For this review, take the finished solid that the model builds, in its own axes (mm). Round coordinates to 2 decimals unless told otherwise and drop trailing zeros. Loops run counter-clockwise (first coordinate to the right, second up) from the corner with the lowest first, then second, coordinate; pieces in that order, holes last. Notation, with made-up numbers: (80.25, 6.5) -> (118.25, 6.5) arc R20 ccw to (118.25, 39.5) -> close; hole circle Ø5 at (72, 47.25). An arc over 180 degrees is marked (long way). Write each question's results on one line, items separated by ' | '.
Autodesk Inventor part; units mm, degrees
ref_plane "YZ Plane" through (0, 0, 0) normal (1, 0, 0) x (0, 1, 0)
ref_plane "XZ Plane" through (0, 0, 0) normal (0, 1, 0) x (-1, 0, 0)
ref_plane "XY Plane" through (0, 0, 0) normal (0, 0, 1) x (1, 0, 0)
sketch "Sketch1" plane through (0, 0, 0) normal (0, 1, 0) x (-1, 0, 0)
  line L0 (0, 0) -> (31, 0)
  line L1 (31, 0) -> (31, -84)
  line L2 (31, -84) -> (0, -84)
  line L3 (0, -84) -> (0, 0)
  line L4 (31, -42) -> (0, -42)
  circle A0 centre (20.5, -3.75) radius 1.5
  circle A1 centre (20.5, -80.25) radius 1.5
  line L5 (15.5, -84) -> (15.5, 0)
  circle A2 centre (25, -42) radius 2
  circle A3 centre (6, -42) radius 2
  dimension "d0" = 84
  dimension "d1" = 31
  dimension "d3" = 3.75
  dimension "d4" = 10.5
  dimension "d5" = 3
  dimension "d7" = 6
  dimension "d8" = 4
extrude "Extrusion1" add sketch "Sketch1" along normal blind 1 contours L0 L5 L4 A3 L3 | L0 L1 L4 A2 L5 | L4 A3 L5 L2 L3 | L4 A2 L1 L2 L5
properties part number "Platte4"
1. Consider section B-B (x = -25). State the section outline as (y, z) points, plus the area to 3 significant figures.
Values found:
outline: (0, -84) -> (1, -84) -> (1, -44) -> (0, -44) -> close; (0, -40) -> (1, -40) -> (1, 0) -> (0, 0) -> close | area: 80.0 mm2
2. Consider section D-D (x = -20.5). State the section outline as (y, z) points, plus the area to 3 significant figures.
Values found:
outline: (0, -84) -> (1, -84) -> (1, -81.75) -> (0, -81.75) -> close; (0, -78.75) -> (1, -78.75) -> (1, -5.25) -> (0, -5.25) -> close; (0, -2.25) -> (1, -2.25) -> (1, 0) -> (0, 0) -> close | area: 78.0 mm2
3. For pin 1 (4 mm diameter, centred on x = -20.5, z = -3.75, fed in from +Y), flat-tipped, find the tip position at first contact; note if it passes through.
Values found:
pin 1: stops at y = 1
4. To check wall thickness, follow probe 1 along X at (y, z) = (0.4, -42); probe 2 along X at (y, z) = (0.55, -40.5); probe 3 along Z at (x, y) = (-25, 0.45). State the ranges of each line that lie inside material, in increasing order.
Values found:
probe 1: x = -31 to -27, -23 to -8, -4 to 0 | probe 2: x = -31 to -26.32, -23.68 to -7.32, -4.68 to 0 | probe 3: z = -84 to -44, -40 to 0
5. Draft analysis for pull direction X (two halves, no side actions). For faces 1 (the face through (-19, 0.5, -3.8)), 2 (the face through (-15, 1, -41)), state which applies: released by +X, released by -X, zero draft, split by the parting line, or undercut.
Values found:
face 1: undercut | face 2: zero draft
6. Consider section A-A (y = 0.25). State the section outline as (x, z) points, plus the area to 3 significant figures.
Values found:
outline: (-31, -84) -> (0, -84) -> (0, 0) -> (-31, 0) -> close; hole circle Ø4 at (-25, -42); hole circle Ø3 at (-20.5, -80.25); hole circle Ø3 at (-20.5, -3.75); hole circle Ø4 at (-6, -42) | area: 2,560 mm2
7. Consider section C-C (z = -80.25). State the section outline as (x, y) points, plus the area to 3 significant figures.
Values found:
outline: (-31, 0) -> (-22, 0) -> (-22, 1) -> (-31, 1) -> close; (-19, 0) -> (0, 0) -> (0, 1) -> (-19, 1) -> close | area: 28.0 mm2
